```python
from build123d import *

# Parameters (mm, degrees)
SKETCH_1_W               = 51
SKETCH_1_H               = 20
EXTRUDE_1_DEPTH          = 20
SKETCH_2_W               = 10
SKETCH_2_H               = 20
CUT_EXTRUDE_1_DEPTH      = 28
SKETCH_3_R               = 4
CUT_EXTRUDE_2_DEPTH      = 1
CUT_EXTRUDE_2_DEPTH_BACK = 52
SKETCH_4_R               = 2
CUT_EXTRUDE_3_DEPTH      = 21


with BuildPart() as part:
    # 草图1 → 凸台-拉伸1 (new body, symmetric)
    with BuildSketch(Plane.XY):
        Rectangle(SKETCH_1_W, SKETCH_1_H)
    extrude(amount=EXTRUDE_1_DEPTH, both=True)

    # 草图2 → 切除-拉伸1 (cut)
    with BuildSketch(Plane.XY.offset(20)):
        Rectangle(SKETCH_2_W, SKETCH_2_H)
    extrude(amount=-CUT_EXTRUDE_1_DEPTH, mode=Mode.SUBTRACT)

    # 草图3 → 切除-拉伸2 (cut, two sides)
    with BuildSketch(Plane.ZY.offset(25.5)) as cut_extrude_2_sk:
        Circle(SKETCH_3_R)
    extrude(amount=CUT_EXTRUDE_2_DEPTH, mode=Mode.SUBTRACT)
    extrude(cut_extrude_2_sk.sketch, amount=-CUT_EXTRUDE_2_DEPTH_BACK, mode=Mode.SUBTRACT)

    # 草图4 → 切除-拉伸3 (cut, through all)
    with BuildSketch(Plane(origin=(0, 10, 0), x_dir=(1, 0, 0), z_dir=(0, 1, 0))):
        with Locations((-22.5, 17)):
            Circle(SKETCH_4_R)
        with Locations((22.5, -17)):
            Circle(SKETCH_4_R)
        with Locations((22.5, 17)):
            Circle(SKETCH_4_R)
        with Locations((-22.5, -17)):
            Circle(SKETCH_4_R)
    extrude(amount=-CUT_EXTRUDE_3_DEPTH, mode=Mode.SUBTRACT)


solid = part.part
```
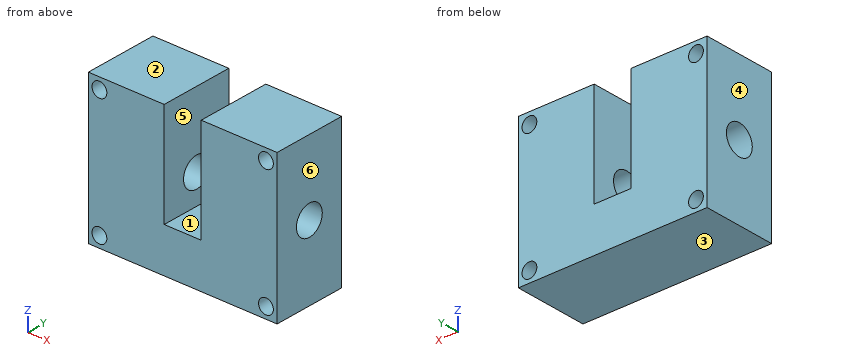
Here's how the part is built. I have some questions about the finished solid (model axes, mm). Face numbers are marked on the shaded views. A direction names the side the tool comes from. Coordinates: 2 decimals unless noted, no trailing zeros. Loops run counter-clockwise (first coordinate to the right, second up) from the corner with the lowest first, then second, coordinate; pieces in that order, holes last. Notation, with made-up numbers: (87.5, 39) - (123.5, 39) arc R22 ccw to (123.5, 53) - close; hole circle Ø5 at (12, -8). An arc over 180 degrees is marked (long way). Return JSON: item names as keys, results as strings. Group by question number.
Item 1: I need wall thicknesses on line 1 (Z direction, x = 22.5, y = 5.75); line 2 (X direction, y = 5.75, z = -17); line 3 (X direction, y = 7, z = -4). Which ranges of each line are inside material? Lowest first, please. Write a range as from..to.
Item 2: If we section it at D-D on z = -17: Write out the boundary of the cut face in (x, y).
Item 3: If we section it at C-C on x = 22.5: Write out the boundary of the cut face in (y, z), and give its area (3 significant figures).
Item 4: On a 3-axis mill with a long thin cutter (end or side, diameter ignored), from which of +Z, -Z, +X, -X, +Y, -Y can I reach the whole of each face in a straight line? I mean the marked faces 1 and 2. Say none if no direction works.
Item 5: We'd pull the mould along X, two halves only. Please class the marked faces 3, 4, 5 and 6: +X half, -X half, draft (parallel to the pull), parting line (faces both ways), or undercut.
Item 6: If we section it at B-B on z = 10: Write out the boundary of the cut face in (x, y), and give its area (3 significant figures).
Item 7: Will this pin go through, and if not, where does the flat tip stop? P1, Ø1.5, axis at x = -2.5, y = 6.5, coming from the +Z side.
Item 8: If we section it at A-A on y = 0: Write out the boundary of the cut face in (x, z).
Calculated:
{
 "1": {"line 1": "z = -20..-19, -15..15, 19..20", "line 2": "x = -25.5..-24.5, -20.5..20.5, 24.5..25.5", "line 3": "x = -25.5..-5, 5..25.5"},
 "2": {"outline": "(-25.5, -10) - (-24.5, -10) - (-24.5, 10) - (-25.5, 10) - close; (-20.5, -10) - (20.5, -10) - (20.5, 10) - (-20.5, 10) - close; (24.5, -10) - (25.5, -10) - (25.5, 10) - (24.5, 10) - close"},
 "3": {"outline": "(-10, -20) - (10, -20) - (10, -19) - (-10, -19) - close; (-10, -15) - (10, -15) - (10, 15) - (-10, 15) - close; (-10, 19) - (10, 19) - (10, 20) - (-10, 20) - close; hole circle Ø8 at (0, 0)", "area": "590 mm^2"},
 "4": {"face 1": "+Z, +Y, -Y", "face 2": "+Z, +X, -X, +Y, -Y"},
 "5": {"face 3": "draft", "face 4": "-X half", "face 5": "undercut", "face 6": "+X half"},
 "6": {"outline": "(-25.5, -10) - (-5, -10) - (-5, 10) - (-25.5, 10) - close; (5, -10) - (25.5, -10) - (25.5, 10) - (5, 10) - close", "area": "820 mm^2"},
 "7": {"P1": "stops at z = -8"},
 "8": {"outline": "(-25.5, -20) - (25.5, -20) - (25.5, -4) - (5, -4) - (5, -8) - (-5, -8) - (-5, -4) - (-25.5, -4) - close; (-25.5, 4) - (-5, 4) - (-5, 20) - (-25.5, 20) - close; (5, 4) - (25.5, 4) - (25.5, 20) - (5, 20) - close; hole circle Ø4 at (-22.5, -17); hole circle Ø4 at (-22.5, 17); hole circle Ø4 at (22.5, -17); hole circle Ø4 at (22.5, 17)"}
}
